Could you check a few things on this model? Use its own coordinates, in mm. Face numbers are marked on the shaded views. A direction names the side the tool comes from. Give positions to 0.01 mm unless a question says otherwise; leave off trailing zeros. Loops run counter-clockwise (first coordinate to the right, second up) from the corner with the lowest first, then second, coordinate; pieces in that order, holes last. Notation, with made-up numbers: M 12,47.5 L 52,47.5 A35 ccw 52,80.5 Z; hole C 40.5,-13.5 d9. An arc over 180 degrees is marked long. Return JSON: item names as keys, results as strings. Group by question number.
1. For pin 1 (5 mm diameter, centred on x = -20.5, z = -42, fed in from -Y); pin 2 (3.5 mm diameter, centred on x = -11.5, y = 14, fed in from +Z); pin 3 (0.9 mm diameter, centred on x = -26.5, y = 13.5, fed in from +Z), each with a flat end and sliding along its axis, tell me the tip position at first contact or that it passes through.
2. If we section it at A-A (x = -18.5): Write out the boundary of the cut face in (y, z).
3. Please list where these lines run through material, in increasing order: line 1 (Z direction, x = -24.5, y = -6.5); line 2 (Y direction, x = -18.5, z = -25.5); line 3 (Y direction, x = -2.75, z = -1.05).
4. For the marked faces 1, 2 and 3, which set-ups out of +Z, -Z, +X, -X, +Y, -Y let a thin tool reach every point of the face, with its end or its side?
5. If we section it at D-D (y = -4.5): Write out the boundary of the cut face in (x, z).
6. If we section it at B-B (y = 7): Write out the boundary of the cut face in (x, z).
7. If we section it at C-C (z = 24): Write out the boundary of the cut face in (x, y).
Autodesk Inventor part; units mm, degrees
ref_plane "YZ Plane" through (0, 0, 0) normal (1, 0, 0) x (0, 1, 0)
ref_plane "XZ Plane" through (0, 0, 0) normal (0, 1, 0) x (-1, 0, 0)
ref_plane "XY Plane" through (0, 0, 0) normal (0, 0, 1) x (1, 0, 0)
sketch "Sketch1" plane through (0, 0, 0) normal (0, 1, 0) x (-1, 0, 0)
  line L0 (0, 0) -> (18.5, 0)
  line L1 (37, 0) -> (37, -25)
  line L2 (0, -25) -> (0, 0)
  line L3 (18.5, -25) -> (18.5, -78)
  line L4 (32.2, -78) -> (32.2, -25)
  line L5 (4.8, -78) -> (4.8, -25)
  line L6 (32.2, -78) -> (4.8, -78)
  line L7 (18.5, -78) -> (18.5, 0)
  line L8 (37, -25) -> (32.2, -25)
  line L9 (18.5, -25) -> (0, -25)
  line L10 (18.5, -25) -> (4.8, -25)
  line L11 (18.5, -78) -> (4.8, -78)
  line L12 (18.5, 0) -> (25.5, 0)
  line L13 (18.5, 0) -> (18.5, 36.8)
  line L14 (18.5, 36.8) -> (18.5, 28.8)
  circle A0 centre (18.5, 28.8) radius 1.5
  dimension "d1" = 25
  dimension "d2" = 53
  dimension "d30" = 36.8
  dimension "d31" = 8
  dimension "d32" = 3
revolve "Revolution1" add sketch "Sketch1" angle 360 about axis through (-18.5, 0, -78) along (0, 0, 1) contours L0 L7 L9 L2 | L3 L6 L5 L9
sketch "Sketch2" plane through (-18.5, 0, 0) normal (0, 0, 1) x (1, 0, 0)
  circle A0 centre (0, 0) radius 15.75
  circle A1 centre (-15.75, 0) radius 1.5
  circle A2 centre (15.75, 0) radius 1.5
  line L0 (0, 0) -> (0, 7)
  circle A3 centre (0, 7) radius 6
  circle A4 centre (0, 7) radius 3
  circle A5 centre (-7.875, 13.6399) radius 1.5
  circle A6 centre (7.875, 13.6399) radius 1.5
  circle A7 centre (-7.875, -13.6399) radius 1.5
  circle A8 centre (7.875, -13.6399) radius 1.5
  point P0 (18.5, 0)
  dimension "d12" = 3
  dimension "d13" = 3
  dimension "d14" = 7
  dimension "d15" = 12
  dimension "d16" = 6
  dimension "d17" = 3
  dimension "d18" = 3
  dimension "d19" = 3
  dimension "d20" = 3
extrude "Extrusion3" add sketch "Sketch2" along normal blind 6.8 contours A3
extrude "Extrusion4" add sketch "Sketch2" along normal blind 36.8 contours A4
extrude "Extrusion5" cut sketch "Sketch2" against normal blind 5 contours A0 A2 | A0 A2 | A6 A0 | A0 A6 | A8 A0 | A0 A8 | A5 A0 | A0 A5 | A7 A0 | A0 A7 | A1 A0 | A0 A1
extrude "Extrusion6" cut sketch "Sketch1" along normal blind 20 contours A0 L13 | L13 A0
properties part number "offcentered_shaft_dc_and_encoder"
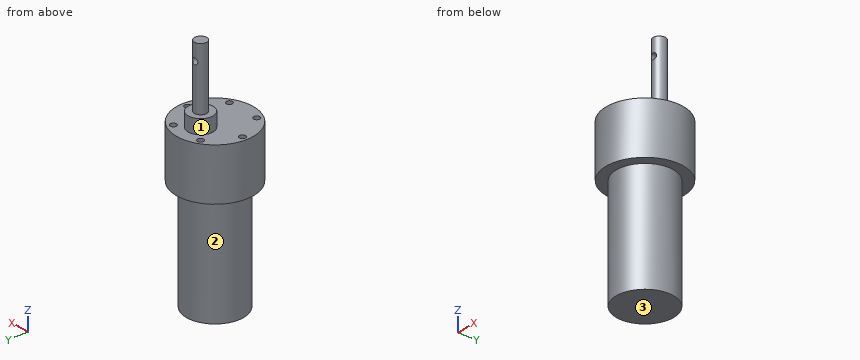
Answer:
{
 "1": {"pin 1": "stops at y = -13.7", "pin 2": "stops at z = 0", "pin 3": "stops at z = -5"},
 "2": {"outline": "M -18.5,-25 L -13.7,-25 L -13.7,-78 L 13.7,-78 L 13.7,-25 L 18.5,-25 L 18.5,0 L 13,0 L 13,6.8 L 10,6.8 L 10,27.3 L 4,27.3 L 4,6.8 L 1,6.8 L 1,0 L -18.5,0 Z; M 4,30.3 L 10,30.3 L 10,36.8 L 4,36.8 Z"},
 "3": {"line 1": "z = -78 to 0", "line 2": "y = -13.7 to 13.7", "line 3": "y = -9.71 to -1.5, 1.5 to 9.71"},
 "4": {"face 1": "+Z", "face 2": "-Z", "face 3": "-Z, +X, -X, +Y, -Y"},
 "5": {"outline": "M -36.44,-25 L -31.44,-25 L -31.44,-78 L -5.56,-78 L -5.56,-25 L -0.56,-25 L -0.56,0 L -36.44,0 Z"},
 "6": {"outline": "M -35.62,-25 L -30.28,-25 L -30.28,-78 L -6.72,-78 L -6.72,-25 L -1.38,-25 L -1.38,0 L -12.5,0 L -12.5,6.8 L -15.5,6.8 L -15.5,36.8 L -21.5,36.8 L -21.5,6.8 L -24.5,6.8 L -24.5,0 L -35.62,0 Z; hole C -18.5,28.8 d3"},
 "7": {"outline": "C -18.5,7 d6"}
}
